Read the model definition and answer for the solid it produces. Units are mm, in the model's axes. Give positions to 0.01 mm unless a question says otherwise; leave off trailing zeros. Order: outer loops, then holes, each group sorted by start corner. A loop starts at its lowest first (then second) coordinate and runs counter-clockwise, first axis right, second up. Notation, with made-up numbers: M 43.25,1.25 L 67.25,1.25 A17 ccw 67.25,24.25 Z; hole C -29,22 d5. An arc over 180 degrees is marked long. One line per item, written item: value. Start each with the question number.
from build123d import *

# Parameters (mm, degrees)
F0_R     = 2
F1_DEPTH = 2.5


with BuildPart() as f1:
    # F0 (on Front) → F1 (new body)
    with BuildSketch(Plane.XZ):
        with BuildLine():
            Line((12.596618, 4), (-12.363835, 3.999805))
            ThreePointArc((-12.363835, 3.999805), (-16.394213, 0.270214), (-12.903364, -3.968625))
            Line((-12.903364, -3.968625), (-11.881677, -3.965836))
            Line((-11.881677, -3.965836), (11.71409, -3.901421))
            Line((11.71409, -3.901421), (13.500497, -3.896544))
            ThreePointArc((13.500497, -3.896544), (16.5707, 0.45489), (12.596618, 4))
        make_face()
        with Locations((-12.40335, 0)):
            Circle(F0_R, mode=Mode.SUBTRACT)
        with BuildLine():
            ThreePointArc((14.59665, 0), (12.59665, -2), (10.59665, 0))
            ThreePointArc((10.59665, 0), (12.59665, 2), (14.59665, 0))
        make_face(mode=Mode.SUBTRACT)
    extrude(amount=F1_DEPTH)


solid = f1.part
Q1. Determine the mould class of faces 1 (the cylindrical face through (-16.39, -1.23, 0.35)), 2 (the cylindrical face through (11.674, -1.232, -1.774)), 3 (the flat face through (0, -2.5, 0)), 4 (the cylindrical face through (-10.496, -1.232, 0.601)) for opening direction Z: released by +Z, released by -Z, zero draft, split by the parting line, or undercut.
Q2. Find section C-C, the plane z = -1.25. Give the vertices of the cut face in (x, y), then the cut area to 3 significant figures.
Q3. Each of these flat-tipped pins is pushed along its axis until it touches: pin 1 (3 mm diameter, centred on x = 11.5, z = -0.5, fed in from +Y); pin 2 (1.5 mm diameter, centred on x = -4, y = -1, fed in from -Z); pin 3 (3 mm diameter, centred on x = 12.6, z = 0, fed in from +Y); pin 4 (1.5 mm diameter, centred on y = -1.5, z = -2.5, fed in from +X). Where does it stop, or does it pass through?
Q4. Find section B-B, the plane y = -0.45. Give the vertices of the cut face in (x, z).
Q5. Find section A-A, the plane z = 0. Give the vertices of the cut face in (x, y).
Q6. Consider probe 1 along X at (y, z) = (-1.1, 1.5); probe 2 along X at (y, z) = (-0.6, -0.5); probe 3 along Z at (x, y) = (13.5, -0.75). Determine where each line is inside the solid, lowest interval first.
Evaluation:
1. face 1: split by the parting line
1. face 2: undercut
1. face 3: zero draft
1. face 4: undercut
2. outline: M -16.2,-2.5 L -13.96,-2.5 L -13.96,0 L -16.2,0 Z; M -10.84,-2.5 L 11.04,-2.5 L 11.04,0 L -10.84,0 Z; M 14.16,-2.5 L 16.4,-2.5 L 16.4,0 L 14.16,0 Z
2. area: 65.9 mm2
3. pin 1: y = 0
3. pin 2: z = -3.95
3. pin 3: through
3. pin 4: x = 16.19
4. outline: M -12.9,-3.97 L -11.88,-3.97 L 11.71,-3.9 L 13.5,-3.9 A4 ccw 12.6,4 L -12.36,4 A4 ccw Z; hole C -12.4,0 d4; hole C 12.6,0 d4
5. outline: M -16.4,-2.5 L -14.4,-2.5 L -14.4,0 L -16.4,0 Z; M -10.4,-2.5 L 10.6,-2.5 L 10.6,0 L -10.4,0 Z; M 14.6,-2.5 L 16.6,-2.5 L 16.6,0 L 14.6,0 Z
6. probe 1: -16.11 to -13.73, -11.08 to 11.27, 13.92 to 16.3
6. probe 2: -16.37 to -14.34, -10.47 to 10.66, 14.53 to 16.57
6. probe 3: -3.9 to -1.78, 1.78 to 3.9
